Read the model definition and answer for the solid it produces. Units are mm, in the model's axes. Face numbers are marked on the shaded views. A direction names the side the tool comes from. Give positions to 0.01 mm unless a question says otherwise; leave off trailing zeros. Write each loop counter-clockwise with the first axis right and the second up, starting at its lowest first coordinate (ties: lowest second). Pieces come first, ordered by that corner, then holes. Notation, with made-up numbers: (39.25, 79.5) - (51.25, 79.5) arc R24 ccw to (51.25, 101.5) - close; hole circle Ø4 at (-25, 69.25). An arc over 180 degrees is marked (long way). Answer as a JSON object with one key per item and string values. Group by question number.
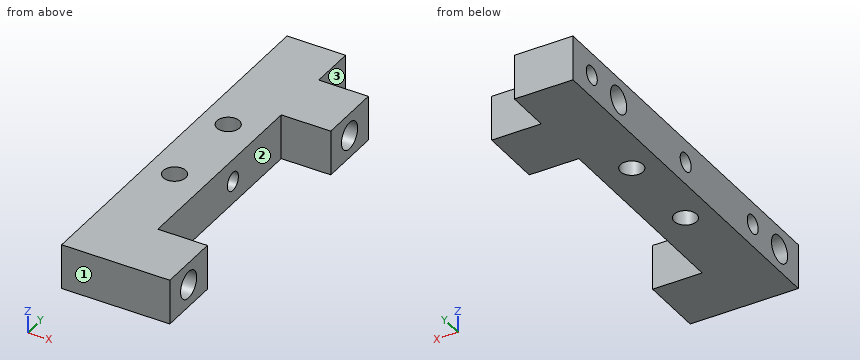
```python
from build123d import *

# Parameters (mm, degrees)
ESQUISSE1_W              = 5
ESQUISSE1_H              = 42
ESQUISSE1_R              = 1.5
EXTRUSION1_DEPTH         = 6
TROU_TARAUD_M3X0_51_D    = 2.5
ESQUISSE4_OUTSIDE_W      = 22.794
ESQUISSE4_OUTSIDE_H      = 52.794
ENL_V_MAT_EXTRU_1_DEPTH  = 23.405356502
TROU_TARAUD_M2_5X0_451_D = 2.05


with BuildPart() as part:
    # Esquisse1 → Extrusion1 (new, symmetric)
    with BuildSketch(Plane(origin=(0, 0, 0), x_dir=(0, 0, -1), z_dir=(1, 0, 0))):
        Rectangle(ESQUISSE1_W, ESQUISSE1_H)
        with Locations((0, -17.5)):
            Circle(ESQUISSE1_R, mode=Mode.SUBTRACT)
        with Locations((0, 12.5)):
            Circle(ESQUISSE1_R, mode=Mode.SUBTRACT)
    extrude(amount=EXTRUSION1_DEPTH, both=True)

    # Trou taraudé M3x0.51 (through all)
    with Locations(Plane(origin=(0, 0, -2.5), x_dir=(-1, 0, 0), z_dir=(0, 0, -1))):
        with Locations((3, 5), (3, -5)):
            Hole(TROU_TARAUD_M3X0_51_D / 2)

    # Esquisse4 outside → Enlèv. mat.-Extru.1 (cut, through all)
    with BuildSketch(Plane(origin=(0, 0, -2.5), x_dir=(-1, 0, 0), z_dir=(0, 0, -1))):
        Rectangle(ESQUISSE4_OUTSIDE_W, ESQUISSE4_OUTSIDE_H)
        Polygon((6, 21), (-0.5, 21), (-0.5, 16), (-6, 16), (-6, 9), (-0.5, 9), (-0.5, -14), (-6, -14), (-6, -21), (6, -21), align=None, mode=Mode.SUBTRACT)
    extrude(amount=-ENL_V_MAT_EXTRU_1_DEPTH, mode=Mode.SUBTRACT)

    # Trou taraudé M2.5x0.451 (through all)
    with Locations(Plane.ZY.offset(6)):
        with Locations((0, 17.5), (0, 0), (0, -12.5)):
            Hole(TROU_TARAUD_M2_5X0_451_D / 2)


solid = part.part
```
1) Find the intervals of material crossed by line 1 (Y direction, x = -1, z = 0) (3 decimals); line 2 (Y direction, x = 1.5, z = 0); line 3 (X direction, y = 7, z = -1.85), in increasing order. Write a range as [from, to].
2) Find section D-D, the plane x = -1.25. Write down the section's boundary in (y, z) (3 decimals), and give its area (3 significant figures).
3) Find section C-C, the plane z = -0.5. Give the number of separate pieces and of enclosed holes in the cut face, and give its area (3 significant figures).
4) Find section B-B, the plane y = 0. Write down the section's boundary in (x, z) (3 decimals), and give its area (3 significant figures).
5) Find section A-A, the plane x = 1.5. Write down the section's boundary in (y, z), and give its area (3 significant figures).
6) Which of the six approach directions +Z, -Z, +X, -X, +Y, -Y give full straight-line access (tool end or side, diameter ignored) to the marked faces 1, 2 and 3?
7) Flat-ended cylindrical pins translate along their axes: pin 1 Ø2.5 at (x, z) = (2, 0.5) entering from +Y; pin 2 Ø2.5 at (y, z) = (-12.5, 0) entering from +X; pin 3 Ø1.6 at (y, z) = (0, 0) entering from +X; pin 4 Ø3 at (x, y) = (-3, 5) entering from -Z. Find the tip coordinate at first contact, or state that the pin passes through.
Values follow:
{
 "1": {"line 1": "y = [-21, -19], [-16, -13.525], [-11.475, -1.025], [1.025, 11], [14, 16.475], [18.525, 21]", "line 2": "y = [-21, -19], [-16, -14], [9, 11], [14, 16]", "line 3": "x = [-6, 0.5]"},
 "2": {"outline": "(-21, -2.5) - (21, -2.5) - (21, 2.5) - (-21, 2.5) - close; hole circle Ø3 at (-17.5, 0); hole circle Ø2.05 at (-12.5, 0); hole circle Ø2.05 at (0, 0); hole circle Ø3 at (12.5, 0); hole circle Ø2.05 at (17.5, 0)", "area": "186 mm2"},
 "3": {"separate pieces": "6", "enclosed holes": "2", "area": "237 mm2"},
 "4": {"outline": "(-6, -2.5) - (0.5, -2.5) - (0.5, -1.025) - (-6, -1.025) - close; (-6, 1.025) - (0.5, 1.025) - (0.5, 2.5) - (-6, 2.5) - close", "area": "19.2 mm2"},
 "5": {"outline": "(-21, -2.5) - (-14, -2.5) - (-14, 2.5) - (-21, 2.5) - close; (9, -2.5) - (16, -2.5) - (16, 2.5) - (9, 2.5) - close; hole circle Ø3 at (-17.5, 0); hole circle Ø3 at (12.5, 0)", "area": "55.9 mm2"},
 "6": {"face 1": "+Z, -Z, +X, -X, -Y", "face 2": "+Z, -Z, +X", "face 3": "+Z, -Z, +X, +Y"},
 "7": {"pin 1": "stops at y = 16", "pin 2": "stops at x = 0.5", "pin 3": "passes through", "pin 4": "stops at z = -2.5"}
}
